For this review, take the finished solid that the model builds, in its own axes (mm). Face numbers are marked on the shaded views. A direction names the side the tool comes from. Round coordinates to 2 decimals unless told otherwise and drop trailing zeros. Loops run counter-clockwise (first coordinate to the right, second up) from the corner with the lowest first, then second, coordinate; pieces in that order, holes last. Notation, with made-up numbers: (70, 42.25) -> (76, 42.25) arc R14 ccw to (76, 59.25) -> close; hole circle Ø11 at (30.25, -15). An arc over 180 degrees is marked (long way). One line per question, with ' | ' between items. Start each with the question number.
1. Consider section A-A (x = 0). Write out the cut boundary in (y, z).
2. Wall thickness on line 1 along Y through (x, z) = (0, 4.25); line 2 along Z through (x, y) = (-2.25, -14); line 3 along Y through (x, z) = (3.5, 3): over which ranges is each line inside the solid? List them lowest first.
3. Draft analysis for pull direction Y (two halves, no side actions). For the marked faces 1, 2, 3 and 4, state which applies: pulls with the +Y half, pulls with the -Y half, needs draft (parallel to the pull), parting line crosses it, or undercut.
4. Consider section D-D (y = -5). Write out the cut boundary in (x, z), and give its area (3 significant figures).
5. Consider section C-C (z = 5.25). Write out the cut boundary in (x, y).
6. For the marked faces 5 and 6, list the 3-axis set-ups (+Z, -Z, +X, -X, +Y, -Y) from which the entire face can be reached by the end or side of a thin tool; tool diameter is ignored.
7. For pin 1 Ø4 at (x, y) = (-2.5, -0.5) entering from +Z; pin 2 Ø3 at (x, y) = (10.5, 8.5) entering from +Z; pin 3 Ø2 at (y, z) = (-7, 6) entering from -X, all flat-tipped, find the tip position at first contact; note any pin that passes through.
8. Consider section B-B (y = 0). Write out the cut boundary in (x, z).
```python
from build123d import *

# Parameters (mm, degrees)
SKETCH_R      = 4
PAD_DEPTH     = 2
SKETCH001_R   = 6.5
SKETCH001_R_2 = 4
PAD001_DEPTH  = 5
CHAMFER_SIZE  = 0.5
FILLET_R      = 3


with BuildPart() as part:
    # Sketch → Pad (new body)
    with BuildSketch(Plane.XY):
        Polygon((0, 16.5), (-14.289419, 8.25), (-14.289419, -8.25), (0, -16.5), (14.289419, -8.25), (14.289419, 8.25), align=None)
        Circle(SKETCH_R, mode=Mode.SUBTRACT)
    extrude(amount=PAD_DEPTH)

    # Sketch001 (on Face9 of Pad) → Pad001 (join)
    with BuildSketch(Plane.XY.offset(2)):
        Circle(SKETCH001_R)
        Circle(SKETCH001_R_2, mode=Mode.SUBTRACT)
    extrude(amount=PAD001_DEPTH)

    # Chamfer
    chamfer_edges = [part.edges().sort_by_distance(p)[0] for p in [
        (-4, 0, 7),
    ]]
    chamfer(chamfer_edges, length=CHAMFER_SIZE)

    # Fillet
    fillet_edges = [part.edges().sort_by_distance(p)[0] for p in [
        (0, -16.5, 1),
        (14.289419, -8.25, 1),
        (14.289419, 8.25, 1),
        (-14.289419, -8.25, 1),
        (-14.289419, 8.25, 1),
        (0, 16.5, 1),
    ]]
    fillet(fillet_edges, radius=FILLET_R)


solid = part.part
```
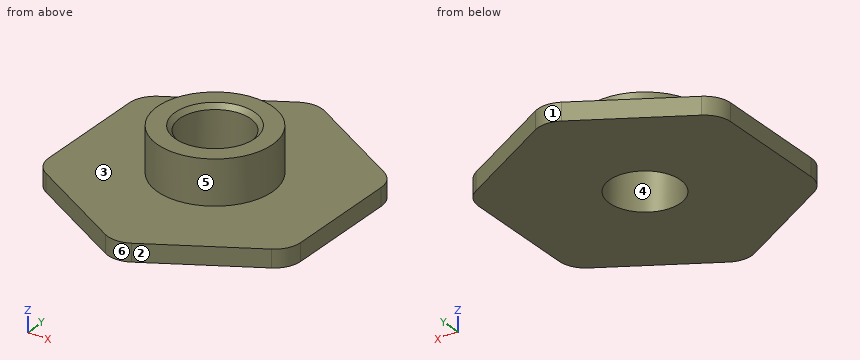
Answer block:
1) outline: (-16.04, 0) -> (-4, 0) -> (-4, 6.5) -> (-4.5, 7) -> (-6.5, 7) -> (-6.5, 2) -> (-16.04, 2) -> close; (4, 0) -> (16.04, 0) -> (16.04, 2) -> (6.5, 2) -> (6.5, 7) -> (4.5, 7) -> (4, 6.5) -> close
2) line 1: y = -6.5 to -4, 4 to 6.5 | line 2: z = 0 to 2 | line 3: y = -5.48 to -1.94, 1.94 to 5.48
3) face 1: pulls with the +Y half | face 2: pulls with the -Y half | face 3: needs draft | face 4: undercut
4) outline: (-14.29, 0) -> (14.29, 0) -> (14.29, 2) -> (4.15, 2) -> (4.15, 7) -> (-4.15, 7) -> (-4.15, 2) -> (-14.29, 2) -> close | area: 98.7 mm2
5) outline: circle Ø13 at (0, 0); hole circle Ø8 at (0, 0)
6) face 5: +Z | face 6: +Z, -Z, -Y
7) pin 1: stops at z = 7 | pin 2: stops at z = 2 | pin 3: stops at x = -2.5
8) outline: (-14.29, 0) -> (-4, 0) -> (-4, 6.5) -> (-4.5, 7) -> (-6.5, 7) -> (-6.5, 2) -> (-14.29, 2) -> close; (4, 0) -> (14.29, 0) -> (14.29, 2) -> (6.5, 2) -> (6.5, 7) -> (4.5, 7) -> (4, 6.5) -> close
